```python
from build123d import *

# Parameters (mm, degrees)
SKETCH1_W           = 100
SKETCH1_H           = 100
BOSS_EXTRUDE1_DEPTH = 46
FILLET1_R           = 6
SHELL1_T            = -3
SKETCH2_R           = 3
SKETCH2_R_2         = 2.25
CUT_EXTRUDE1_DEPTH  = 10
SKETCH3_W           = 26
SKETCH3_H           = 56
SKETCH3_W_2         = 20
SKETCH3_H_2         = 50
BOSS_EXTRUDE2_DEPTH = 5
SKETCH4_R           = 2.5
SKETCH4_R_2         = 1.25
SKETCH4_R_3         = 3
BOSS_EXTRUDE3_DEPTH = 6
SKETCH5_R           = 9
CUT_EXTRUDE2_DEPTH  = 6
SKETCH6_R           = 6
SKETCH6_R_2         = 1.25
BOSS_EXTRUDE4_DEPTH = 8
SKETCH7_R           = 2.75
BOSS_EXTRUDE5_DEPTH = 6
CHAMFER1_SIZE       = 2
FILLET2_R           = 2


with BuildPart() as part:
    # Sketch1 → Boss-Extrude1 (new body)
    with BuildSketch(Plane.XY):
        Rectangle(SKETCH1_W, SKETCH1_H)
    extrude(amount=BOSS_EXTRUDE1_DEPTH)

    # Fillet1
    fillet1_edges = [part.edges().sort_by_distance(p)[0] for p in [
        (50, -50, 23),
        (-50, -50, 23),
        (-50, 50, 23),
        (50, 50, 23),
    ]]
    fillet(fillet1_edges, radius=FILLET1_R)

    # Shell1
    shell1_openings = [part.faces().sort_by_distance(p)[0] for p in [
        (0, 0, 46),
    ]]
    offset(amount=SHELL1_T, openings=shell1_openings, kind=Kind.INTERSECTION)

    # Sketch2 → Cut-Extrude1 (cut)
    with BuildSketch(Plane(origin=(50, 0, 0), x_dir=(0, 0, -1), z_dir=(1, 0, 0))):
        with Locations(Location((-34, 35, 0), (0, 0, 90))):
            Circle(SKETCH2_R)
        with Locations(Location((-34, -35, 0), (0, 0, 90))):
            Circle(SKETCH2_R)
        with Locations(Location((-12, -35, 0), (0, 0, 90))):
            Circle(SKETCH2_R)
        with Locations(Location((-12, 35, 0), (0, 0, 90))):
            Circle(SKETCH2_R_2)
    extrude(amount=-CUT_EXTRUDE1_DEPTH, mode=Mode.SUBTRACT)

    # Sketch3 → Boss-Extrude2 (add)
    with BuildSketch(Plane.XY.offset(3)):
        with Locations((27, 2)):
            Rectangle(SKETCH3_W, SKETCH3_H)
        with Locations((27, 2)):
            Rectangle(SKETCH3_W_2, SKETCH3_H_2, mode=Mode.SUBTRACT)
    extrude(amount=BOSS_EXTRUDE2_DEPTH)

    # Sketch4 → Boss-Extrude3 (add)
    # profile 1 of 4: a face of its own
    with BuildSketch(Plane.XY.offset(3)):
        with Locations((-25.81005519, 37)):
            Circle(SKETCH4_R)
        with Locations((-25.81005519, 37)):
            Circle(SKETCH4_R_2, mode=Mode.SUBTRACT)
    # profile 2 of 4: a face of its own
    with BuildSketch(Plane.XY.offset(3)):
        with Locations((2.12994481, 37)):
            Circle(SKETCH4_R)
        with Locations((2.12994481, 37)):
            Circle(SKETCH4_R_2, mode=Mode.SUBTRACT)
    # profile 3 of 4: a face of its own
    with BuildSketch(Plane.XY.offset(3)):
        with Locations((7.03, -15.07)):
            Circle(SKETCH4_R)
        with Locations((7.03, -15.07)):
            Circle(SKETCH4_R_2, mode=Mode.SUBTRACT)
    # profile 4 of 4: a face of its own
    with BuildSketch(Plane.XY.offset(3)):
        with Locations((-41.05005519, -13.8)):
            Circle(SKETCH4_R_3)
        with Locations((-41.05005519, -13.8)):
            Circle(SKETCH4_R_2, mode=Mode.SUBTRACT)
    extrude(amount=BOSS_EXTRUDE3_DEPTH)

    # Sketch5 → Cut-Extrude2 (cut)
    with BuildSketch(Plane.XZ.offset(50)):
        with Locations(Location((-30, 17, 0), (0, 0, 270))):
            Circle(SKETCH5_R)
    extrude(amount=-CUT_EXTRUDE2_DEPTH, mode=Mode.SUBTRACT)

    # Sketch6 → Boss-Extrude4 (add)
    # profile 1 of 4: a face of its own
    with BuildSketch(Plane.XY.offset(46)):
        with Locations((44, 44)):
            Circle(SKETCH6_R)
        with Locations((44, 44)):
            Circle(SKETCH6_R_2, mode=Mode.SUBTRACT)
    # profile 2 of 4: a face of its own
    with BuildSketch(Plane.XY.offset(46)):
        with Locations((44, -44)):
            Circle(SKETCH6_R)
        with Locations((44, -44)):
            Circle(SKETCH6_R_2, mode=Mode.SUBTRACT)
    # profile 3 of 4: a face of its own
    with BuildSketch(Plane.XY.offset(46)):
        with Locations((-44, -44)):
            Circle(SKETCH6_R)
        with Locations((-44, -44)):
            Circle(SKETCH6_R_2, mode=Mode.SUBTRACT)
    # profile 4 of 4: a face of its own
    with BuildSketch(Plane.XY.offset(46)):
        with Locations((-44, 44)):
            Circle(SKETCH6_R)
        with Locations((-44, 44)):
            Circle(SKETCH6_R_2, mode=Mode.SUBTRACT)
    extrude(amount=-BOSS_EXTRUDE4_DEPTH)

    # Sketch7 → Boss-Extrude5 (add)
    # profile 1 of 2: a face of its own
    with BuildSketch(Plane(origin=(0, 0, 0), x_dir=(-1, 0, 0), z_dir=(0, 0, -1))):
        with BuildLine():
            Line((-50, 10), (-64, 10))
            ThreePointArc((-64, 10), (-68.242640687, 8.242640687), (-70, 4))
            Line((-70, 4), (-70, -4))
            ThreePointArc((-70, -4), (-68.242640687, -8.242640687), (-64, -10))
            Line((-64, -10), (-50, -10))
            Line((-50, -10), (-50, 10))
        make_face()
        with Locations((-60, 0)):
            Circle(SKETCH7_R, mode=Mode.SUBTRACT)
    # profile 2 of 2: a face of its own
    with BuildSketch(Plane(origin=(0, 0, 0), x_dir=(-1, 0, 0), z_dir=(0, 0, -1))):
        with BuildLine():
            Line((70, 4), (70, -4))
            ThreePointArc((70, -4), (68.242640687, -8.242640687), (64, -10))
            Line((64, -10), (50, -10))
            Line((50, -10), (50, 10))
            Line((50, 10), (64, 10))
            ThreePointArc((64, 10), (68.242640687, 8.242640687), (70, 4))
        make_face()
        with Locations(Location((60, 0, 0), (0, 0, 180))):
            Circle(SKETCH7_R, mode=Mode.SUBTRACT)
    extrude(amount=-BOSS_EXTRUDE5_DEPTH)

    # Chamfer1
    chamfer1_edges = [part.edges().sort_by_distance(p)[0] for p in [
        (62.75, 0, 6),
        (-62.75, 0, 6),
    ]]
    chamfer(chamfer1_edges, length=CHAMFER1_SIZE)

    # Fillet2
    fillet2_edges = [part.edges().sort_by_distance(p)[0] for p in [
        (38.803847577, 47, 42),
        (47, 38.803847577, 42),
        (38.803847577, -47, 42),
        (47, -38.803847577, 42),
        (-38.803847577, -47, 42),
        (-47, -38.803847577, 42),
        (-47, 38.803847577, 42),
        (-38.803847577, 47, 42),
        (50, 0, 6),
        (-50, 0, 6),
    ]]
    fillet(fillet2_edges, radius=FILLET2_R)


solid = part.part
```
Geometry: final body of the model. Coordinates: model frame, mm. A direction names the side the tool comes from. Coordinates: 2 decimals unless noted, no trailing zeros. Order: outer loops, then holes, each group sorted by start corner. A loop starts at its lowest first (then second) coordinate and runs counter-clockwise, first axis right, second up.
Item 1: Section query C-C (x = -30). Output: boundary loops of the cut face in (y, z).
Answer:
outline: (-50, 0) - (50, 0) - (50, 46) - (47, 46) - (47, 3) - (-47, 3) - (-47, 8) - (-50, 8) - close; (-50, 26) - (-47, 26) - (-47, 46) - (-50, 46) - close
Item 2: Access query for faces 4 (the face through (-57, -10, 3)), 5 (the face through (1.59, 34.56, 5.96)), 6 (the face through (46.14, 46.1, 20.74)). Directions: +Z, -Z, +X, -X, +Y, -Y. A direction counts if a zero-diameter tool reaches every point of the face in a straight line with its end or side. Return the directions, or none.
Answer:
face 4: +Z, -Z, -X, -Y
face 5: +Z
face 6: none
Item 3: Material intervals for line 1 along Y through (x, z) = (44, 42); line 2 along Y through (x, z) = (-8, 22.5), sorted ascending.
Answer:
line 1: y = -50 to -45.25, -42.75 to -38, 38 to 42.75, 45.25 to 50
line 2: y = -50 to -47, 47 to 50
Item 4: Section query A-A (y = 0). State how many separate pieces and enclosed holes the cut face has, then the cut area to 3 significant figures.
Answer:
separate pieces: 3
enclosed holes: 0
area: 756 mm2
Item 5: Draft query along X for faces 1 (the face through (48.521, 36.21, 13.897)), 2 (the face through (-44.047, -13.668, 5.958)), 3 (the face through (-48.289, -48.196, 23.322)). Return one class per face: released by +X, released by -X, zero draft, split by the parting line, or undercut.
Answer:
face 1: zero draft
face 2: undercut
face 3: released by -X
Item 6: Contact query for flat-ended pins moving along their axis: P1, Ø12, axis at y = 1.5, z = 32, coming from the -X side; P2, Ø10, axis at x = 31, y = -38.5, coming from the +Z side; P3, Ø21.5, axis at y = -14.5, z = 32, coming from the +X side. Output: stop coordinate, or through.
Answer:
P1: stops at x = -50
P2: stops at z = 3
P3: stops at x = 50
Item 7: Section query D-D (x = 60). Output: boundary loops of the cut face in (y, z), then the cut area to 3 significant figures.
Answer:
outline: (-10, 0) - (-2.75, 0) - (-2.75, 4) - (-4.75, 6) - (-10, 6) - close; (2.75, 0) - (10, 0) - (10, 6) - (4.75, 6) - (2.75, 4) - close
area: 83.0 mm2
Item 8: Section query B-B (z = 34). Output: boundary loops of the cut face in (x, y).
Answer:
outline: (-50, -44) arc R6 ccw to (-44, -50) - (44, -50) arc R6 ccw to (50, -44) - (50, -38) - (47, -38) - (47, -44) arc R3 cw to (44, -47) - (-44, -47) arc R3 cw to (-47, -44) - (-47, 44) arc R3 cw to (-44, 47) - (44, 47) arc R3 cw to (47, 44) - (47, 38) - (50, 38) - (50, 44) arc R6 ccw to (44, 50) - (-44, 50) arc R6 ccw to (-50, 44) - close; (47, -32) - (50, -32) - (50, 32) - (47, 32) - close
